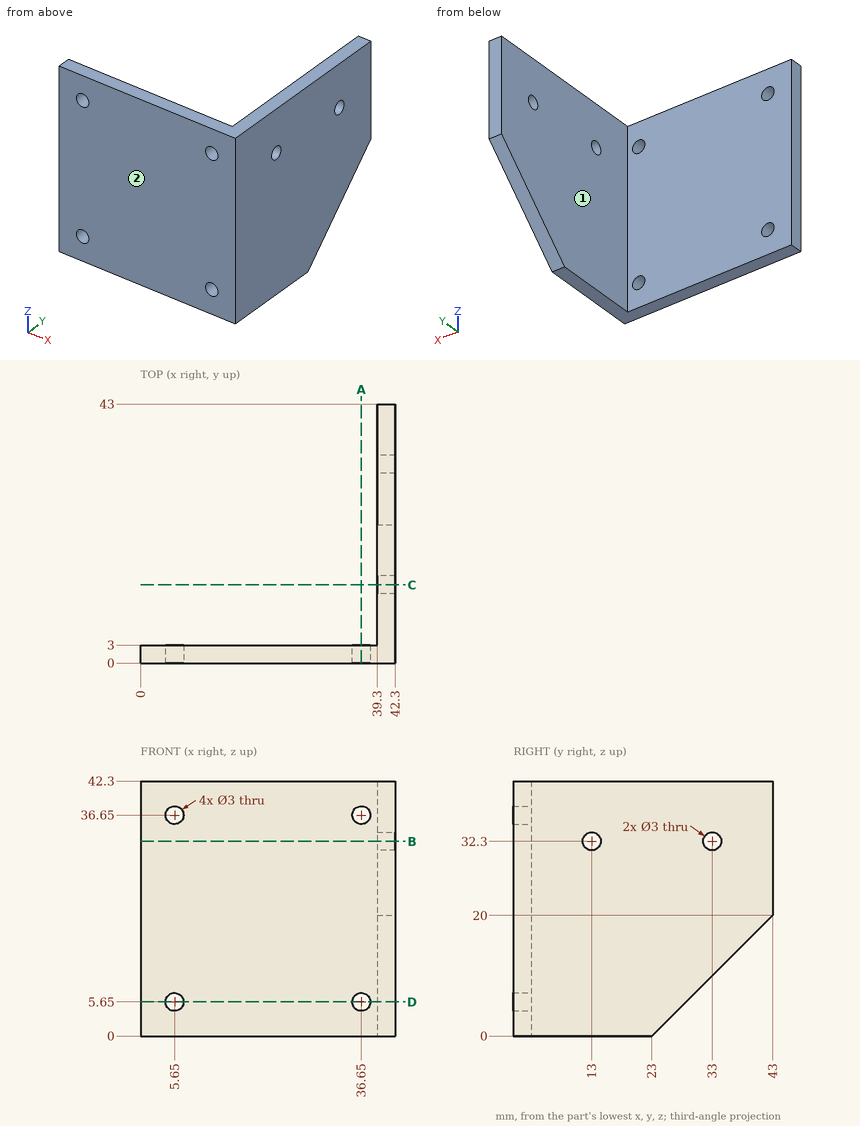
Print and shaded views of the part. All mm, measured from the part's lowest x, y and z. A direction names the side the tool comes from. Round coordinates to 2 decimals unless told otherwise and drop trailing zeros. Write each loop counter-clockwise with the first axis right and the second up, starting at its lowest first coordinate (ties: lowest second). Pieces come first, ordered by that corner, then holes. Notation, with made-up numbers: (-17.75, 67) -> (37.25, 67) arc R11 cw to (37.25, 71) -> close; hole circle Ø11 at (51, 7). An arc over 180 degrees is marked (long way). Return JSON: item names as keys, results as strings. Group by question number.
Q1. Probe L1, parallel to X at y = 1.25, z = 36.65; L2, parallel to Y at x = 41, z = 32. List the from-to ranges inside material, lowest first. Write a range as [from, to].
Q2. Saw through at C-C on y = 13. Write the cut outline in (x, z), plus the area to 3 significant figures.
Q3. Saw through at D-D on z = 5.65. Write the cut outline in (x, y).
Q4. Pin check, flat tip, straight feed: pin 1 (6 mm diameter, centred on x = 32.5, z = 28.5, fed in from +Y). Stop position of the tip, or through.
Q5. Saw through at B-B on z = 32.3. Write the cut outline in (x, y), plus the area to 3 significant figures.
Q6. Saw through at A-A on x = 36.65. Write the cut outline in (y, z), plus the area to 3 significant figures.
Q7. Which spindle directions (+Z, -Z, +X, -X, +Y, -Y) get a long thin tool onto all of the face, cutting with end or side? Do the marked faces 1 and 2. Say none if no direction does.
Answer:
{
 "1": {"L1": "[0, 4.15], [7.15, 35.15], [38.15, 42.3]", "L2": "[0, 11.53], [14.47, 31.53], [34.47, 43]"},
 "2": {"outline": "(39.3, 0) -> (42.3, 0) -> (42.3, 30.8) -> (39.3, 30.8) -> close; (39.3, 33.8) -> (42.3, 33.8) -> (42.3, 42.3) -> (39.3, 42.3) -> close", "area": "118 mm2"},
 "3": {"outline": "(0, 0) -> (4.15, 0) -> (4.15, 3) -> (0, 3) -> close; (7.15, 0) -> (35.15, 0) -> (35.15, 3) -> (7.15, 3) -> close; (38.15, 0) -> (42.3, 0) -> (42.3, 28.65) -> (39.3, 28.65) -> (39.3, 3) -> (38.15, 3) -> close"},
 "4": {"pin 1": "y = 3"},
 "5": {"outline": "(0, 0) -> (42.3, 0) -> (42.3, 11.5) -> (39.3, 11.5) -> (39.3, 3) -> (0, 3) -> close; (39.3, 14.5) -> (42.3, 14.5) -> (42.3, 31.5) -> (39.3, 31.5) -> close; (39.3, 34.5) -> (42.3, 34.5) -> (42.3, 43) -> (39.3, 43) -> close", "area": "229 mm2"},
 "6": {"outline": "(0, 0) -> (3, 0) -> (3, 4.15) -> (0, 4.15) -> close; (0, 7.15) -> (3, 7.15) -> (3, 35.15) -> (0, 35.15) -> close; (0, 38.15) -> (3, 38.15) -> (3, 42.3) -> (0, 42.3) -> close", "area": "109 mm2"},
 "7": {"face 1": "+Z, -Z, -X, +Y", "face 2": "+Z, -Z, +X, -X, -Y"}
}
